Work out the finished part from the listing and answer in its coordinate system (mm). A direction names the side the tool comes from. Coordinates: 2 decimals unless noted, no trailing zeros. Loops run counter-clockwise (first coordinate to the right, second up) from the corner with the lowest first, then second, coordinate; pieces in that order, holes last. Notation, with made-up numbers: (17.25, 34) -> (26.25, 34) arc R16 ccw to (26.25, 56) -> close; hole circle Ø10 at (35, 7.5). An arc over 180 degrees is marked (long way). Use a Markdown table: item, result. Add a question column.
```python
from build123d import *

# Parameters (mm, degrees)
F0_W      = 65
F0_H      = 80
F1_DEPTH  = 35
F2_R      = 5
F3_T      = -1.5
F6_DEPTH  = 8
F7_R      = 2.5
F7_R_2    = 1.375
F9_DEPTH  = 5
F10_W     = 6
F10_H     = 7.5
F11_DEPTH = 8
F12_SIZE  = 5.99999


# Not quite as in the source:
# - a fillet or chamfer is up to 0.001 mm smaller than in the source, because OpenCascade refuses the exact size


with BuildPart() as f1:
    # F0 (on Top) → F1 (new body)
    with BuildSketch(Plane.XY):
        with Locations((1.2058935761, -13.8313528726)):
            Rectangle(F0_W, F0_H)
    extrude(amount=F1_DEPTH)

    # F2
    f2_edges = [f1.edges().sort_by_distance(p)[0] for p in [
        (-31.294106, -53.831353, 17.5),
        (-31.294106, 26.168647, 17.5),
        (33.705894, -53.831353, 17.5),
        (33.705894, 26.168647, 17.5),
    ]]
    fillet(f2_edges, radius=F2_R)

    # F3
    f3_openings = [f1.faces().sort_by_distance(p)[0] for p in [
        (1.205894, -13.831353, 35),
    ]]
    offset(amount=F3_T, openings=f3_openings)

    # F5 (on offset) → F6 (join)
    with BuildSketch(Plane.XY.offset(33.5)):
        with BuildLine():
            Line((-29.7941064239, 18.6686471274), (-23.7941064239, 18.6686471274))
            Line((-23.7941064239, 18.6686471274), (-23.7941064239, 24.6686471274))
            Line((-23.7941064239, 24.6686471274), (-26.2941064239, 24.6686471274))
            ThreePointArc((-26.2941064239, 24.6686471274), (-28.768980158, 23.6435208615), (-29.7941064239, 21.1686471274))
            Line((-29.7941064239, 21.1686471274), (-29.7941064239, 18.6686471274))
        make_face()
        with BuildLine():
            Line((28.7058935761, 24.6686471274), (26.2058935761, 24.6686471274))
            Line((26.2058935761, 24.6686471274), (26.2058935761, 18.6686471274))
            Line((26.2058935761, 18.6686471274), (32.2058935761, 18.6686471274))
            Line((32.2058935761, 18.6686471274), (32.2058935761, 21.1686471274))
            ThreePointArc((32.2058935761, 21.1686471274), (31.1807673103, 23.6435208615), (28.7058935761, 24.6686471274))
        make_face()
        with BuildLine():
            Line((26.2058935761, -46.3313528726), (26.2058935761, -52.3313528726))
            Line((26.2058935761, -52.3313528726), (28.7058935761, -52.3313528726))
            ThreePointArc((28.7058935761, -52.3313528726), (31.1807673103, -51.3062266068), (32.2058935761, -48.8313528726))
            Line((32.2058935761, -48.8313528726), (32.2058935761, -46.3313528726))
            Line((32.2058935761, -46.3313528726), (26.2058935761, -46.3313528726))
        make_face()
        with BuildLine():
            Line((-23.7941064239, -46.3313528726), (-29.7941064239, -46.3313528726))
            Line((-29.7941064239, -46.3313528726), (-29.7941064239, -48.8313528726))
            ThreePointArc((-29.7941064239, -48.8313528726), (-28.768980158, -51.3062266068), (-26.2941064239, -52.3313528726))
            Line((-26.2941064239, -52.3313528726), (-23.7941064239, -52.3313528726))
            Line((-23.7941064239, -52.3313528726), (-23.7941064239, -46.3313528726))
        make_face()
    extrude(amount=-F6_DEPTH)

    # F7 (on face) → F9 (join)
    with BuildSketch(Plane.XY.offset(1.5)):
        with Locations((-22.5441064239, 13.6686471274)):
            Circle(F7_R)
        with Locations((-22.5441064239, 13.6686471274)):
            Circle(F7_R_2, mode=Mode.SUBTRACT)
        with Locations((-22.5441064239, -8.3313528726)):
            Circle(F7_R)
        with Locations((-22.5441064239, -8.3313528726)):
            Circle(F7_R_2, mode=Mode.SUBTRACT)
        with Locations((24.9558935761, 13.6686471274)):
            Circle(F7_R)
        with Locations((24.9558935761, 13.6686471274)):
            Circle(F7_R_2, mode=Mode.SUBTRACT)
        with Locations((24.9558935761, -8.3313528726)):
            Circle(F7_R)
        with Locations((24.9558935761, -8.3313528726)):
            Circle(F7_R_2, mode=Mode.SUBTRACT)
        with BuildLine():
            Line((17.2198255986, -40.3313528726), (21.6919615536, -40.3313528726))
            ThreePointArc((21.6919615536, -40.3313528726), (22.258410653, -39.4018191419), (22.4558935761, -38.3313528726))
            ThreePointArc((22.4558935761, -38.3313528726), (18.3854273068, -35.5288357957), (17.2198255986, -40.3313528726))
        make_face()
        with BuildLine():
            ThreePointArc((-14.0441064239, -38.3313528726), (-18.1145726932, -35.5288357957), (-19.2801744014, -40.3313528726))
            Line((-19.2801744014, -40.3313528726), (-14.8080384464, -40.3313528726))
            ThreePointArc((-14.8080384464, -40.3313528726), (-14.241589347, -39.4018191419), (-14.0441064239, -38.3313528726))
        make_face()
    extrude(amount=F9_DEPTH)

    # F10 (on offset) → F11 (join)
    with BuildSketch(Plane.XY.offset(20)):
        with Locations((5.2058935761, 22.4186471274)):
            Rectangle(F10_W, F10_H)
        with BuildLine():
            Line((26.2058935761, 18.6686471274), (32.2058935761, 18.6686471274))
            Line((32.2058935761, 18.6686471274), (32.2058935761, 21.1686471274))
            ThreePointArc((32.2058935761, 21.1686471274), (31.1807673103, 23.6435208615), (28.7058935761, 24.6686471274))
            Line((28.7058935761, 24.6686471274), (26.2058935761, 24.6686471274))
            Line((26.2058935761, 24.6686471274), (26.2058935761, 18.6686471274))
        make_face()
        with BuildLine():
            Line((32.2058935761, -46.3313528726), (26.2058935761, -46.3313528726))
            Line((26.2058935761, -46.3313528726), (26.2058935761, -52.3313528726))
            Line((26.2058935761, -52.3313528726), (28.7058935761, -52.3313528726))
            ThreePointArc((28.7058935761, -52.3313528726), (31.1807673103, -51.3062266068), (32.2058935761, -48.8313528726))
            Line((32.2058935761, -48.8313528726), (32.2058935761, -46.3313528726))
        make_face()
        with Locations((5.2058935761, -50.0813528726)):
            Rectangle(F10_W, F10_H)
    extrude(amount=-F11_DEPTH)

    # F12 (size 6 in the source; OpenCascade refuses exactly that, so slightly less here)
    f12_edges = [f1.edges().sort_by_distance(p)[0] for p in [
        (29.205894, -46.331353, 25.5),
        (29.205894, -46.331353, 12),
        (5.205894, -46.331353, 12),
        (29.205894, 18.668647, 12),
        (29.205894, 18.668647, 25.5),
        (5.205894, 18.668647, 12),
        (-26.794106, 18.668647, 25.5),
        (-26.794106, -46.331353, 25.5),
    ]]
    chamfer(f12_edges, length=F12_SIZE)


solid = f1.part
```
Item 1: Section B-B (y = -43.5) is taken. Determine the outline of the cut face in (x, z).
Item 2: For faces 1 (the face through (-26.84, 21.63, 28.54)), 2 (the face through (32.2, -52.41, 17.74)), 3 (the face through (23.113, 15.358, 3.965)), determine the directions among +Z, -Z, +X, -X, +Y, -Y from which every point of the face is accessible in a straight line to the end or side of a thin tool.
Item 3: Section A-A (z = 3) is taken. Count the separate pieces of the cut face and the enclosed holes in it, then the cut area to 3 significant figures.
Item 4: For a pull along X with two mould halves and no side action, classify faces 4 (the face through (1, -53.831, 17)), 5 (the face through (26.206, -50, 17)), 6 (the face through (33.706, -14, 17)) as +X half, -X half, draft (parallel to the pull), parting line (faces both ways), or undercut.
Item 5: Section C-C (z = 23) is taken. Determine the outline of the cut face in (x, y).
Item 6: Given pin 1 (2 mm diameter, centred on x = 6.5, y = -17.5, fed in from +Z); pin 2 (2.5 mm diameter, centred on x = 18, y = -37, fed in from +Z); pin 3 (2 mm diameter, centred on x = -24, y = -22, fed in from -Z); pin 4 (1.8 mm diameter, centred on x = -25.5, y = 23, fed in from +Z), each flat-ended and moving along its own axis, determine where each tip first touches the part or whether it passes through.
Item 7: Find the intervals of material crossed by probe 1 along X at (y, z) = (-1.5, 4); probe 2 along Y at (x, z) = (4, 26); probe 3 along Z at (x, y) = (27, 11), in increasing order.
Item 8: Section D-D (x = 12) is taken. Determine the outline of the cut face in (y, z).
Output:
| question | item | result |
|---|---|---|
| 1 | outline | (-31.29, 0) -> (33.71, 0) -> (33.71, 35) -> (32.21, 35) -> (32.21, 1.5) -> (-29.79, 1.5) -> (-29.79, 35) -> (-31.29, 35) -> close |
| 2 | face 1 | none |
| 2 | face 2 | +Z, -Z, +X, -Y |
| 2 | face 3 | +Z |
| 3 | separate pieces | 7 |
| 3 | enclosed holes | 5 |
| 3 | area | 520 mm2 |
| 4 | face 4 | draft |
| 4 | face 5 | undercut |
| 4 | face 6 | +X half |
| 5 | outline | (-31.29, -48.83) arc R5 ccw to (-26.29, -53.83) -> (28.71, -53.83) arc R5 ccw to (33.71, -48.83) -> (33.71, 21.17) arc R5 ccw to (28.71, 26.17) -> (-26.29, 26.17) arc R5 ccw to (-31.29, 21.17) -> close; hole (-29.79, -48.83) arc R3.5 ccw to (-26.29, -52.33) -> (28.71, -52.33) arc R3.5 ccw to (32.21, -48.83) -> (32.21, 21.17) arc R3.5 ccw to (28.71, 24.67) -> (-26.29, 24.67) arc R3.5 ccw to (-29.79, 21.17) -> close |
| 6 | pin 1 | stops at z = 1.5 |
| 6 | pin 2 | stops at z = 6.5 |
| 6 | pin 3 | stops at z = 0 |
| 6 | pin 4 | stops at z = 33.5 |
| 7 | probe 1 | x = -31.29 to -29.79, 32.21 to 33.71 |
| 7 | probe 2 | y = -53.83 to -52.33, 24.67 to 26.17 |
| 7 | probe 3 | z = 0 to 1.5 |
| 8 | outline | (-53.83, 0) -> (26.17, 0) -> (26.17, 35) -> (24.67, 35) -> (24.67, 1.5) -> (-52.33, 1.5) -> (-52.33, 35) -> (-53.83, 35) -> close |
